```python
from build123d import *

# Parameters (mm, degrees)
SKETCH1_R                = 19.01
SKETCH1_R_2              = 13.5
BOSS_EXTRUDE1_DEPTH      = 18
BOSS_EXTRUDE2_DEPTH      = 23
BOSS_EXTRUDE2_DEPTH_BACK = 18
SKETCH2_R                = 21
SKETCH2_R_2              = 13.5
CUT_EXTRUDE1_DEPTH       = 13
MIRROR2_COPY_1_DEPTH     = 13
BOSS_EXTRUDE3_START      = -5
SKETCH4_W                = 6
SKETCH4_H                = 8
SKETCH4_R                = 2
BOSS_EXTRUDE3_DEPTH      = 5.0001
FILLET1_R                = 2
FILLET1_OF_MIRROR5_R     = 2
BOSS_EXTRUDE6_START      = 0.0001
SKETCH7_W                = 6
SKETCH7_H                = 8
SKETCH7_R                = 2
BOSS_EXTRUDE6_DEPTH      = 5.0001
FILLET2_R                = 2
CUT_EXTRUDE2_START       = -0.0001
SKETCH9_R                = 1.5
CUT_EXTRUDE2_DEPTH       = 20.0001


with BuildPart() as part:
    # Sketch1 → Boss-Extrude1 (new body)
    with BuildSketch(Plane.XY):
        Circle(SKETCH1_R)
        Circle(SKETCH1_R_2, mode=Mode.SUBTRACT)
    extrude(amount=BOSS_EXTRUDE1_DEPTH)

    # Sketch2 → Boss-Extrude2 (add, two sides: drawn at the far end of the back side and taken through both)
    with BuildSketch(Plane.XY.offset(18).offset(-BOSS_EXTRUDE2_DEPTH_BACK)):
        Circle(SKETCH2_R)
        Circle(SKETCH2_R_2, mode=Mode.SUBTRACT)
    extrude(amount=BOSS_EXTRUDE2_DEPTH + BOSS_EXTRUDE2_DEPTH_BACK)

    # Sketch3 → Cut-Extrude1 (cut)
    with BuildSketch(Plane(origin=(0, 0, 0), x_dir=(-1, 0, 0), z_dir=(0, 0, -1))):
        Polygon((15.540276616, 12.01617991), (10.937752349, 10.062524267), (14.845063634, 0.857475733), (19.447587901, 2.811131375), align=None)
    cut_extrude1 = extrude(amount=-CUT_EXTRUDE1_DEPTH, mode=Mode.SUBTRACT)

    # Mirror1: Cut-Extrude1 across plane
    add(cut_extrude1.mirror(Plane.ZX), mode=Mode.SUBTRACT)

    # Mirror2: Cut-Extrude1 across plane
    add(cut_extrude1.mirror(Plane(origin=(0, 0, 0), x_dir=(0, 0, 1), z_dir=(1, 0, 0))), mode=Mode.SUBTRACT)

    # Mirror2 copy 1 sketch → Mirror2 copy 1 (cut)
    with BuildSketch(Plane(origin=(0, 0, 0), x_dir=(1, 0, 0), z_dir=(0, 0, -1))):
        Polygon((15.540276616, 12.01617991), (10.937752349, 10.062524267), (14.845063634, 0.857475733), (19.447587901, 2.811131375), align=None)
    extrude(amount=-MIRROR2_COPY_1_DEPTH, mode=Mode.SUBTRACT)

    # Sketch4 → Boss-Extrude3 (add)
    with BuildSketch(Plane(origin=(0, 0, 0), x_dir=(-1, 0, 0), z_dir=(0, 0, -1)).offset(BOSS_EXTRUDE3_START)):
        with Locations((0, 24)):
            Rectangle(SKETCH4_W, SKETCH4_H)
        with Locations((0, 24)):
            Circle(SKETCH4_R, mode=Mode.SUBTRACT)
    boss_extrude3 = extrude(amount=BOSS_EXTRUDE3_DEPTH)

    # Fillet1
    fillet1_edges = [part.edges().sort_by_distance(p)[0] for p in [
        (-3, 28, 2.49995),
        (3, 28, 2.49995),
    ]]
    fillet(fillet1_edges, radius=FILLET1_R)

    # Mirror5: Boss-Extrude3 across plane
    add(boss_extrude3.mirror(Plane.ZX))

    # Fillet1 of Mirror5
    fillet1_of_mirror5_edges = [part.edges().sort_by_distance(p)[0] for p in [
        (-3, -28, 2.49995),
        (3, -28, 2.49995),
    ]]
    fillet(fillet1_of_mirror5_edges, radius=FILLET1_OF_MIRROR5_R)

    # Sketch7 → Boss-Extrude6 (add)
    with BuildSketch(Plane.XY.offset(41).offset(BOSS_EXTRUDE6_START)):
        with Locations((0, 24)):
            Rectangle(SKETCH7_W, SKETCH7_H)
        with Locations(Location((0, 24, 0), (0, 0, 180))):
            Circle(SKETCH7_R, mode=Mode.SUBTRACT)
    boss_extrude6 = extrude(amount=-BOSS_EXTRUDE6_DEPTH)

    # Mirror6: Boss-Extrude6 across plane
    add(boss_extrude6.mirror(Plane.ZX))

    # Fillet2
    fillet2_edges = [part.edges().sort_by_distance(p)[0] for p in [
        (-3, 28, 38.50005),
        (3, 28, 38.50005),
        (-3, -28, 38.50005),
        (3, -28, 38.50005),
    ]]
    fillet(fillet2_edges, radius=FILLET2_R)

    # Sketch9 → Cut-Extrude2 (cut)
    with BuildSketch(Plane(origin=(0, 0, 0), x_dir=(1, 0, 0), z_dir=(0, 1, 0)).offset(CUT_EXTRUDE2_START)):
        with Locations(Location((-8.25, -31, 0), (0, 0, 90))):
            Circle(SKETCH9_R)
    cut_extrude2 = extrude(amount=CUT_EXTRUDE2_DEPTH, mode=Mode.SUBTRACT)

    # Mirror7: Cut-Extrude2 across plane
    add(cut_extrude2.mirror(Plane(origin=(0, 0, 0), x_dir=(0, 0, 1), z_dir=(1, 0, 0))), mode=Mode.SUBTRACT)


solid = part.part
```
Could you check a few things on this model? Use its own coordinates, in mm. A direction names the side the tool comes from. Round coordinates to 2 decimals unless told otherwise and drop trailing zeros. Order: outer loops, then holes, each group sorted by start corner. A loop starts at its lowest first (then second) coordinate and runs counter-clockwise, first axis right, second up. Notation, with made-up numbers: M 13.5,-26.5 L 49.5,-26.5 A21 ccw 49.5,-15.5 Z; hole C 1.25,20.25 d1. An arc over 180 degrees is marked long. One line per question, with ' | ' between items. Start each with the question number.
(1) Suppose I cut it at C-C on z = 11.5. List the corners of the cut face in (x, y) for me, then the cut area to 3 significant figures.
(2) Thinking about a two-plate mould opening in X: for faces 4 (the face through (-1, 22, 41)), 5 (the face through (3, -24, 39)), 6 (the face through (-13.271, -11.053, 6.409)), which applies, +X half, -X half, draft (parallel to the pull), parting line (faces both ways), or undercut?
(3) Please list where these lines run through material, in increasing order: line 1 along Y through (x, z) = (0, 1.8); line 2 along Z through (x, y) = (8.25, 15.75); line 3 along Z through (x, y) = (1.5, 21).
(4) Suppose I cut it at B-B on x = 7.5. List the corners of the cut face in (y, z) for me.
(5) Suppose I cut it at D-D on y = 0. List the corners of the cut face in (x, z) for me, then the cut area to 3 significant figures.
(6) For faces 1 (the face through (17.11, -1.82, 6.41)), 2 (the face through (-9.26, 14.54, 32.11)), 3 (the face through (0, -28, 39)), which set-ups out of +Z, -Z, +X, -X, +Y, -Y let a thin tool reach every point of the face, with its end or its side?
(7) Suppose I cut it at A-A on y = -24. List the corners of the cut face in (x, z) for me.
(8) For P1, Ø2.5, axis at x = 8.25, z = 31, coming from the +Y side; P2, Ø1.5, axis at y = -23.5, z = 1.5, coming from the +X side; P3, Ø4, axis at y = 24, z = 38.5, coming from the -X side, each with a flat end and sliding along its axis, tell me the tip position at first contact or that it passes through.
Geometry results:
1) outline: C 0,0 d42; hole M -19.45,-2.81 L -15.54,-12.02 L -10.94,-10.06 L -14.85,-0.86 Z; hole M -19.45,2.81 L -14.85,0.86 L -10.94,10.06 L -15.54,12.02 Z; hole C 0,0 d27; hole M 10.94,-10.06 L 15.54,-12.02 L 19.45,-2.81 L 14.85,-0.86 Z; hole M 10.94,10.06 L 14.85,0.86 L 19.45,2.81 L 15.54,12.02 Z | area: 613 mm²
2) face 4: draft | face 5: +X half | face 6: undercut
3) line 1: -28 to -26, -22 to -13.5, 13.5 to 22, 26 to 28 | line 2: 0 to 29.5, 32.5 to 41 | line 3: 0 to 5, 36 to 41
4) outline: M -19.62,0 L -11.22,0 L -11.22,41 L -19.62,41 Z; M 11.22,0 L 19.62,0 L 19.62,29.7 L 11.22,29.7 Z; M 11.22,32.3 L 19.62,32.3 L 19.62,41 L 11.22,41 Z
5) outline: M -21,0 L -13.5,0 L -13.5,41 L -21,41 Z; M 13.5,0 L 21,0 L 21,41 L 13.5,41 Z | area: 615 mm²
6) face 1: -Z | face 2: +Y | face 3: +Z, -Z, +X, -X, -Y
7) outline: M -3,0 L -2,0 L -2,5 L -3,5 Z; M -3,36 L -2,36 L -2,41 L -3,41 Z; M 2,0 L 3,0 L 3,5 L 2,5 Z; M 2,36 L 3,36 L 3,41 L 2,41 Z
8) P1: y = -9.59 | P2: x = 3 | P3: x = -3
